Could you check a few things on this model? Use its own coordinates, in mm. Give positions to 0.01 mm unless a question says otherwise; leave off trailing zeros. Write each loop counter-clockwise with the first axis right and the second up, starting at its lowest first coordinate (ties: lowest second). Pieces come first, ordered by that corner, then holes. Notation, with made-up numbers: (-11, -26) - (43, -26) arc R26 cw to (43, 9) - close; hole circle Ø5 at (30, -8). An arc over 180 degrees is marked (long way). Answer as CSV lines item,"result". Start each with the question number.
Q1. Imagine slicing it at A-A on y = 4.25. List the corners of the cut face in (x, z) for me.
Q2. Imagine slicing it at C-C on y = 8. List the corners of the cut face in (x, z) for me, and give its area (3 significant figures).
Q3. If I drill on line 1 along X through (y, z) = (6.25, 0); line 2 along X through (y, z) = (15.5, -0.1); line 3 along Y through (x, z) = (0.9, 0.2), over which ranges is the centre line in solid material (lowest first)?
Q4. Will this pin go through, and if not, where does the flat tip stop? pin 1 Ø1 at (x, z) = (2, -1) entering from -Y.
Q5. Imagine slicing it at B-B on z = 0. List the corners of the cut face in (x, y) for me, and give its area (3 significant figures).
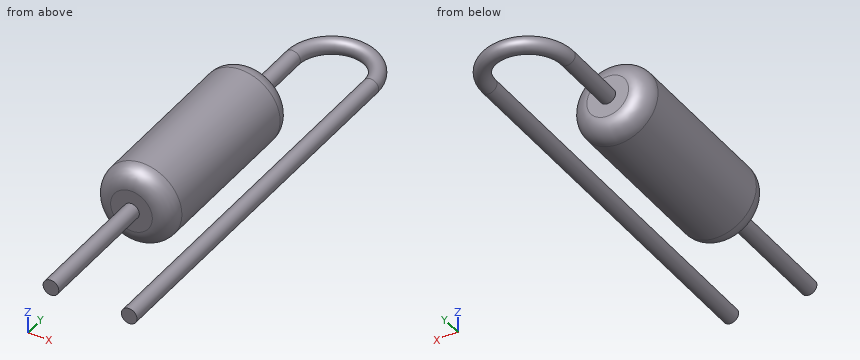
```python
from build123d import *

# Parameters (mm, degrees)
SKETCH_2_R      = 0.3
SKETCH_3_R      = 1.5
EXTRUDE_1_DEPTH = 7.5
FILLET_1_R      = 0.7


with BuildPart() as part:
    # По траектории1: sweep along a path in Эскиз1
    with BuildLine(Plane.XY) as sweep_1_path:
        Line((0, 0), (0, 15))
        ThreePointArc((0, 15), (1.5, 16.5), (3, 15))
        Line((3, 15), (3, 0))
    # Эскиз2 → По траектории1 (sweep)
    with BuildSketch(Plane(origin=(0, 0, 0), x_dir=(1, 0, 0), z_dir=(0, 1, 0))):
        Circle(SKETCH_2_R)
    sweep(path=sweep_1_path.line)

    # Эскиз3 → Вытянуть1 (add)
    with BuildSketch(Plane.XZ.offset(-5)):
        with Locations(Location((0, 0, 0), (0, 0, 270))):
            Circle(SKETCH_3_R)
    extrude(amount=-EXTRUDE_1_DEPTH)

    # Скругление1
    fillet_1_edges = [part.edges().sort_by_distance(p)[0] for p in [
        (0, 5, 1.5),
        (0, 12.5, 1.5),
    ]]
    fillet(fillet_1_edges, radius=FILLET_1_R)


solid = part.part
```
Conclusion:
1,outline,"circle Ø0.6 at (0, 0); circle Ø0.6 at (3, 0)"
2,outline,"circle Ø3 at (0, 0); circle Ø0.6 at (3, 0)"
2,area,"7.35 mm^2"
3,line 1,"-1.5 to 1.5, 2.7 to 3.3"
3,line 2,"-0.21 to 0.39, 2.61 to 3.21"
3,line 3,"5.01 to 12.49, 16.13 to 16.62"
4,pin 1,"through"
5,outline,"(-1.5, 5.7) arc R0.7 ccw to (-0.8, 5) - (-0.3, 5) - (-0.3, 0) - (0.3, 0) - (0.3, 5) - (0.8, 5) arc R0.7 ccw to (1.5, 5.7) - (1.5, 11.8) arc R0.7 ccw to (0.8, 12.5) - (0.3, 12.5) - (0.3, 15) arc R1.2 cw to (2.7, 15) - (2.7, 0) - (3.3, 0) - (3.3, 15) arc R1.8 ccw to (-0.3, 15) - (-0.3, 12.5) - (-0.8, 12.5) arc R0.7 ccw to (-1.5, 11.8) - close"
5,area,"38.4 mm^2"
